```python
from build123d import *

# Parameters (mm, degrees)
SKETCH1_W           = 304.8
SKETCH1_H           = 304.8
SKETCH1_R           = 3.175
SKETCH1_R_2         = 3.2639
BOSS_EXTRUDE1_DEPTH = 3.175


with BuildPart() as part:
    # Sketch1 → Boss-Extrude1 (new body)
    with BuildSketch(Plane.XY):
        Rectangle(SKETCH1_W, SKETCH1_H)
        with Locations((-101.6, 0)):
            Circle(SKETCH1_R, mode=Mode.SUBTRACT)
        with Locations((-50.8, 0)):
            Circle(SKETCH1_R, mode=Mode.SUBTRACT)
        Circle(SKETCH1_R, mode=Mode.SUBTRACT)
        with Locations((101.6, 0)):
            Circle(SKETCH1_R, mode=Mode.SUBTRACT)
        with Locations((50.8, 0)):
            Circle(SKETCH1_R, mode=Mode.SUBTRACT)
        with Locations((-50.8, 127)):
            Circle(SKETCH1_R, mode=Mode.SUBTRACT)
        with Locations((0, 127)):
            Circle(SKETCH1_R, mode=Mode.SUBTRACT)
        with Locations((50.8, 127)):
            Circle(SKETCH1_R, mode=Mode.SUBTRACT)
        with Locations((-101.6, 72.39)):
            Circle(SKETCH1_R, mode=Mode.SUBTRACT)
        with Locations((0, 72.39)):
            Circle(SKETCH1_R, mode=Mode.SUBTRACT)
        with Locations((101.6, 72.39)):
            Circle(SKETCH1_R, mode=Mode.SUBTRACT)
        with Locations((-101.6, -72.39)):
            Circle(SKETCH1_R, mode=Mode.SUBTRACT)
        with Locations((0, -72.39)):
            Circle(SKETCH1_R, mode=Mode.SUBTRACT)
        with Locations((101.6, -72.39)):
            Circle(SKETCH1_R, mode=Mode.SUBTRACT)
        with Locations((50.8, -127)):
            Circle(SKETCH1_R, mode=Mode.SUBTRACT)
        with Locations((0, -127)):
            Circle(SKETCH1_R, mode=Mode.SUBTRACT)
        with Locations((-50.8, -127)):
            Circle(SKETCH1_R, mode=Mode.SUBTRACT)
        with Locations((-101.6, 97.79)):
            Circle(SKETCH1_R, mode=Mode.SUBTRACT)
        with Locations((0, 97.79)):
            Circle(SKETCH1_R, mode=Mode.SUBTRACT)
        with Locations((101.6, 97.79)):
            Circle(SKETCH1_R, mode=Mode.SUBTRACT)
        with Locations((101.6, 127)):
            Circle(SKETCH1_R, mode=Mode.SUBTRACT)
        with Locations((-101.6, 127)):
            Circle(SKETCH1_R, mode=Mode.SUBTRACT)
        with Locations((-118.11, 33.02)):
            Circle(SKETCH1_R, mode=Mode.SUBTRACT)
        with Locations((-101.6, -127)):
            Circle(SKETCH1_R, mode=Mode.SUBTRACT)
        with Locations((101.6, -127)):
            Circle(SKETCH1_R, mode=Mode.SUBTRACT)
        with Locations((101.6, -97.79)):
            Circle(SKETCH1_R, mode=Mode.SUBTRACT)
        with Locations((0, -97.79)):
            Circle(SKETCH1_R, mode=Mode.SUBTRACT)
        with Locations((-101.6, -97.79)):
            Circle(SKETCH1_R, mode=Mode.SUBTRACT)
        with Locations((-118.11, -33.02)):
            Circle(SKETCH1_R, mode=Mode.SUBTRACT)
        with Locations((-139.7, 139.7)):
            Circle(SKETCH1_R_2, mode=Mode.SUBTRACT)
        with Locations((-139.7, 0)):
            Circle(SKETCH1_R_2, mode=Mode.SUBTRACT)
        with Locations((-139.7, -139.7)):
            Circle(SKETCH1_R_2, mode=Mode.SUBTRACT)
        with Locations((139.7, -139.7)):
            Circle(SKETCH1_R_2, mode=Mode.SUBTRACT)
        with Locations((139.7, 0)):
            Circle(SKETCH1_R_2, mode=Mode.SUBTRACT)
        with Locations((139.7, 139.7)):
            Circle(SKETCH1_R_2, mode=Mode.SUBTRACT)
        with Locations((118.11, 33.02)):
            Circle(SKETCH1_R, mode=Mode.SUBTRACT)
        with Locations((118.11, -33.02)):
            Circle(SKETCH1_R, mode=Mode.SUBTRACT)
        with BuildLine():
            Line((-95.25, 125.4125), (-95.25, 128.5875))
            ThreePointArc((-95.25, 128.5875), (-76.2, 147.6375), (-57.15, 128.5875))
            Line((-57.15, 128.5875), (-57.15, 125.4125))
            ThreePointArc((-57.15, 125.4125), (-76.2, 106.3625), (-95.25, 125.4125))
        make_face(mode=Mode.SUBTRACT)
        with BuildLine():
            Line((-6.35, 125.4125), (-6.35, 128.5875))
            ThreePointArc((-6.35, 128.5875), (-25.4, 147.6375), (-44.45, 128.5875))
            Line((-44.45, 128.5875), (-44.45, 125.4125))
            ThreePointArc((-44.45, 125.4125), (-25.4, 106.3625), (-6.35, 125.4125))
        make_face(mode=Mode.SUBTRACT)
        with BuildLine():
            Line((6.35, 125.4125), (6.35, 128.5875))
            ThreePointArc((6.35, 128.5875), (25.4, 147.6375), (44.45, 128.5875))
            Line((44.45, 128.5875), (44.45, 125.4125))
            ThreePointArc((44.45, 125.4125), (25.4, 106.3625), (6.35, 125.4125))
        make_face(mode=Mode.SUBTRACT)
        with BuildLine():
            Line((95.25, 125.4125), (95.25, 128.5875))
            ThreePointArc((95.25, 128.5875), (76.2, 147.6375), (57.15, 128.5875))
            Line((57.15, 128.5875), (57.15, 125.4125))
            ThreePointArc((57.15, 125.4125), (76.2, 106.3625), (95.25, 125.4125))
        make_face(mode=Mode.SUBTRACT)
        with BuildLine():
            Line((-95.25, -125.4125), (-95.25, -128.5875))
            ThreePointArc((-95.25, -128.5875), (-76.2, -147.6375), (-57.15, -128.5875))
            Line((-57.15, -128.5875), (-57.15, -125.4125))
            ThreePointArc((-57.15, -125.4125), (-76.2, -106.3625), (-95.25, -125.4125))
        make_face(mode=Mode.SUBTRACT)
        with BuildLine():
            Line((-6.35, -125.4125), (-6.35, -128.5875))
            ThreePointArc((-6.35, -128.5875), (-25.4, -147.6375), (-44.45, -128.5875))
            Line((-44.45, -128.5875), (-44.45, -125.4125))
            ThreePointArc((-44.45, -125.4125), (-25.4, -106.3625), (-6.35, -125.4125))
        make_face(mode=Mode.SUBTRACT)
        with BuildLine():
            Line((6.35, -125.4125), (6.35, -128.5875))
            ThreePointArc((6.35, -128.5875), (25.4, -147.6375), (44.45, -128.5875))
            Line((44.45, -128.5875), (44.45, -125.4125))
            ThreePointArc((44.45, -125.4125), (25.4, -106.3625), (6.35, -125.4125))
        make_face(mode=Mode.SUBTRACT)
        with BuildLine():
            Line((95.25, -125.4125), (95.25, -128.5875))
            ThreePointArc((95.25, -128.5875), (76.2, -147.6375), (57.15, -128.5875))
            Line((57.15, -128.5875), (57.15, -125.4125))
            ThreePointArc((57.15, -125.4125), (76.2, -106.3625), (95.25, -125.4125))
        make_face(mode=Mode.SUBTRACT)
    extrude(amount=BOSS_EXTRUDE1_DEPTH)


solid = part.part
```
Geometry check sheet. Reference: the model listing, model coordinates, mm. Coordinates: 2 decimals unless noted, no trailing zeros. Write each loop counter-clockwise with the first axis right and the second up, starting at its lowest first coordinate (ties: lowest second). Pieces come first, ordered by that corner, then holes. Notation, with made-up numbers: M 1.25,33 L 8.25,33 A15 ccw 8.25,50 Z; hole C -3.75,-38 d6. An arc over 180 degrees is marked long. Use one line per item in the form item = value. Start each with the question number.
1) Section check B-B on y = -115. Enter the section's corners in (x, z) (1 decimal), and give its area (3 significant figures).
2) Section check A-A on x = 25.4. Enter the section's corners in (y, z) (1 decimal), and give its area (3 significant figures).
3) Section check C-C on z = 2.2. State how many separate pieces and enclosed holes the cut face has, and give its area (3 significant figures).
4) Section check D-D on x = 90.5. Enter the section's corners in (y, z) (3 decimals).
5) Release check for a two-part mould opening along X. For faces 1 (the flat face through (32, 2, 3.175)), 2 (the cylindrical face through (25.819, -106.367, 1.565)) record: pulls with the +X half, pulls with the -X half, needs draft (parallel to the pull), parting line crosses it, or undercut.
6) Thickness scan on probe 1 along Y at (x, z) = (118.11, 2.05) (3 decimals); probe 2 along Y at (x, z) = (-50.8, 2.5) (3 decimals); probe 3 along Y at (x, z) = (-85, 1.25). Record the ranges inside material, lowest first. Write a range as from..to.
Responses:
q1.outline = M -152.4,0 L -92.2,0 L -92.2,3.2 L -152.4,3.2 Z; M -60.2,0 L -41.4,0 L -41.4,3.2 L -60.2,3.2 Z; M -9.4,0 L 9.4,0 L 9.4,3.2 L -9.4,3.2 Z; M 41.4,0 L 60.2,0 L 60.2,3.2 L 41.4,3.2 Z; M 92.2,0 L 152.4,0 L 152.4,3.2 L 92.2,3.2 Z
q1.area = 563 mm2
q2.outline = M -152.4,0 L -147.6,0 L -147.6,3.2 L -152.4,3.2 Z; M -106.4,0 L 106.4,0 L 106.4,3.2 L -106.4,3.2 Z; M 147.6,0 L 152.4,0 L 152.4,3.2 L 147.6,3.2 Z
q2.area = 706 mm2
q3.separate_pieces = 1
q3.enclosed_holes = 45
q3.area = 81,600 mm2
q4.outline = M -152.4,0 L -141.174,0 L -141.174,3.175 L -152.4,3.175 Z; M -112.826,0 L 112.826,0 L 112.826,3.175 L -112.826,3.175 Z; M 141.174,0 L 152.4,0 L 152.4,3.175 L 141.174,3.175 Z
q5.face_1 = needs draft
q5.face_2 = undercut
q6.probe_1 = -152.4..-36.195, -29.845..29.845, 36.195..152.4
q6.probe_2 = -152.4..-130.175, -123.825..-3.175, 3.175..123.825, 130.175..152.4
q6.probe_3 = -152.4..-145.48, -108.52..108.52, 145.48..152.4
